```python
from build123d import *

# Parameters (mm, degrees)
PAD_DEPTH   = 37
THICKNESS_T = -2
SKETCH002_R = 3
HOLE_DEPTH  = 25
HOLE_TIPS_R = 3
FILLET_R    = 3


with BuildPart() as part:
    # Sketch001 → Pad (new body)
    with BuildSketch(Plane.XY):
        with BuildLine():
            Line((-58, 21.65), (56, 21.65))
            Line((56, 21.65), (56, -21.65))
            Line((56, -21.65), (-58, -21.65))
            add(Edge.make_bspline(
                [(-58, -21.65), (-93, -21.65), (-93, -5)],
                knots=[0, 0, 0, 1, 1, 1], degree=2))
            Line((-93, -5), (-93, 5))
            add(Edge.make_bspline(
                [(-58, 21.65), (-93, 21.65), (-93, 5)],
                knots=[0, 0, 0, 1, 1, 1], degree=2))
        make_face()
    extrude(amount=PAD_DEPTH)

    # Thickness
    thickness_openings = [part.faces().sort_by_distance(p)[0] for p in [
        (-16.404598, 0, 37),
        (-16.404598, 0, 0),
    ]]
    offset(amount=THICKNESS_T, openings=thickness_openings)

    # Sketch002 (on Face5 of Thickness) → Hole (cut)
    with BuildSketch(Plane(origin=(-93, 0, 0), x_dir=(0, -1, 0), z_dir=(-1, 0, 0))):
        with Locations((0, 20)):
            Circle(SKETCH002_R)
    extrude(amount=-HOLE_DEPTH, mode=Mode.SUBTRACT)

    # Hole tips → Hole tip 1 section 0
    with BuildSketch(Plane(origin=(-68, 0, 0), x_dir=(0, -1, 0), z_dir=(-1, 0, 0)), mode=Mode.PRIVATE) as hole_tip_1_s0:
        with Locations((0, 20)):
            Circle(HOLE_TIPS_R)
    loft([hole_tip_1_s0.sketch, Vertex(-66.197418, 0, 20)], mode=Mode.SUBTRACT)

    # Fillet
    fillet_edges = [part.edges().sort_by_distance(p)[0] for p in [
        (56, 21.65, 18.5),
        (56, -21.65, 18.5),
    ]]
    fillet(fillet_edges, radius=FILLET_R)


solid = part.part
```
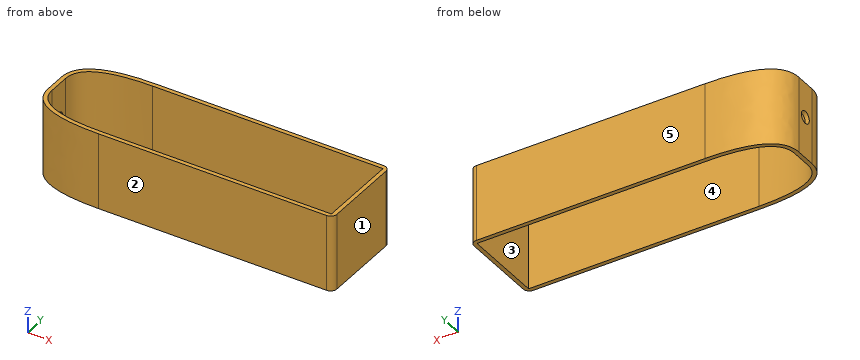
Geometry check sheet. Reference: the model listing, model coordinates, mm. Face numbers are marked on the shaded views. A direction names the side the tool comes from. Coordinates: 2 decimals unless noted, no trailing zeros. Loops run counter-clockwise (first coordinate to the right, second up) from the corner with the lowest first, then second, coordinate; pieces in that order, holes last.
Item 1: Release check for a two-part mould opening along X. For the marked faces 1, 2 and 3 record: released by +X, released by -X, zero draft, split by the parting line, or undercut.
Item 2: Thickness scan on line 1 (Z direction, x = -91.9, y = 0); line 2 (Y direction, x = -9, z = 15.5); line 3 (X direction, y = 1, z = 28). Record the ranges inside material, lowest first.
Item 3: Sectioned sample at A-A, the plane x = 29.5. Record the boundary of the cut face in (y, z), then the cut area to 3 significant figures.
Item 4: Access from +Z, -Z, +X, -X, +Y, -Y to the whole of each face (thin tool, end or side, straight path). Record for the marked faces 4 and 5.
Item 5: Sectioned sample at B-B, the plane y = 0. Record the boundary of the cut face in (x, z), then the cut area to 3 significant figures.
Item 6: Go/stop test with a flat-tipped pin: pin 1 Ø10 at (y, z) = (-11, 13.5) entering from -X. Record where the tip stops, or that it passes through.
Check result:
1. face 1: released by +X
1. face 2: zero draft
1. face 3: undercut
2. line 1: z = 0 to 17, 23 to 37
2. line 2: y = -21.65 to -19.65, 19.65 to 21.65
2. line 3: x = -93 to -91, 54 to 56
3. outline: (-21.65, 0) - (-19.65, 0) - (-19.65, 37) - (-21.65, 37) - close; (19.65, 0) - (21.65, 0) - (21.65, 37) - (19.65, 37) - close
3. area: 148 mm2
4. face 4: +Z, -Z
4. face 5: +Z, -Z, +X, -X, +Y
5. outline: (-93, 0) - (-91, 0) - (-91, 17) - (-93, 17) - close; (-93, 23) - (-91, 23) - (-91, 37) - (-93, 37) - close; (54, 0) - (56, 0) - (56, 37) - (54, 37) - close
5. area: 136 mm2
6. pin 1: stops at x = -92.97
